Check sheet for the modelled part. Datum: model origin and axes. Units: mm. Coordinates: 2 decimals unless noted, no trailing zeros. Write each loop counter-clockwise with the first axis right and the second up, starting at its lowest first coordinate (ties: lowest second). Pieces come first, ordered by that corner, then holes. Notation, with made-up numbers: (79, 66) -> (92, 66) arc R23 ccw to (92, 77) -> close; hole circle Ø11 at (38, -27.5). An arc over 180 degrees is marked (long way). Put each result on its own line as item: value.
```python
from build123d import *

# Parameters (mm, degrees)
BLOCO_DEPTH            = 9.2
ESBO_O3_W              = 5.6
ESBO_O3_H              = 3.2
RASGO_DO_ENCAIXE_DEPTH = 18.034534118


with BuildPart() as part:
    # Esboço1 → Bloco (new body)
    with BuildSketch(Plane(origin=(0, 0, 0), x_dir=(1, 0, 0), z_dir=(0, 1, 0))):
        with BuildLine():
            Line((0, -75), (0.029321703, -68))
            Line((0.029321703, -68), (-12.770566003, -67.946383642))
            Line((-12.770566003, -67.946383642), (-12.795506441, -73.900439883))
            ThreePointArc((-12.795506441, -73.900439883), (-6.421331979, -74.724604352), (0, -75))
        make_face()
    extrude(amount=BLOCO_DEPTH)

    # Esboço3 → Rasgo do Encaixe (cut, through all)
    with BuildSketch(Plane(origin=(-0.284833888, 0, 67.99868406), x_dir=(-0.9999912270311377, 0, -0.0041887779553967395), z_dir=(0.0041887779553967395, 0, -0.9999912270311377))):
        with Locations((2.485841653, 1.6)):
            Rectangle(ESBO_O3_W, ESBO_O3_H)
    extrude(amount=-RASGO_DO_ENCAIXE_DEPTH, mode=Mode.SUBTRACT)


solid = part.part
```
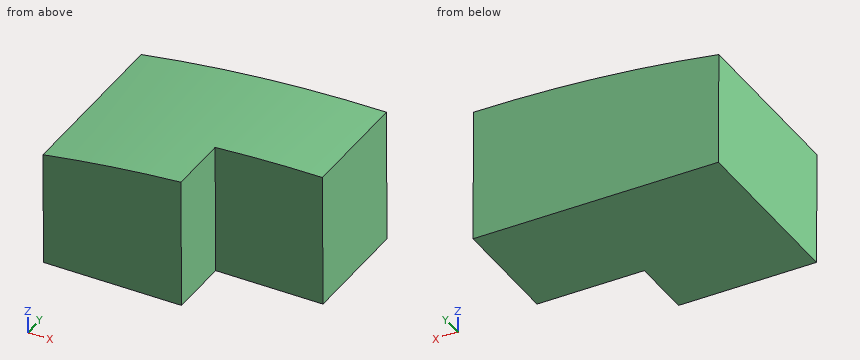
Q1. Cross-section at D-D (z = 70.75). Record the cut outline in (x, y), plus the area to 3 significant figures.
Recorded:
outline: (-12.78, 0) -> (-5.58, 0) -> (-5.58, 3.2) -> (0.02, 3.2) -> (0.02, 9.2) -> (-12.78, 9.2) -> close
area: 99.8 mm2
Q2. Cross-section at C-C (x = -9.25). Record the cut outline in (y, z).
Recorded:
outline: (0, 67.96) -> (9.2, 67.96) -> (9.2, 74.43) -> (0, 74.43) -> close
Q3. Depth check by flat-ended pin: P1, Ø1.7, axis at x = -2.5, z = 70, coming from the -Y side; P2, Ø4, axis at y = 2, z = 74, coming from the +X side; P3, Ø1.5, axis at x = -6, y = 6, coming from the +Z side. Enter the tip coordinate at first touch or a pass-through.
Recorded:
P1: stops at y = 3.2
P2: stops at x = 0.01
P3: stops at z = 74.82
Q4. Material ranges on line 1 along X through (y, z) = (7.5, 68.75); line 2 along Y through (x, z) = (-2.25, 69.25); line 3 along Z through (x, y) = (-9, 1.75), recorded low to high.
Recorded:
line 1: x = -12.77 to 0.03
line 2: y = 3.2 to 9.2
line 3: z = 67.96 to 74.46
Q5. Cross-section at B-B (y = 2.25). Record the cut outline in (x, z).
Recorded:
outline: (-12.8, 73.9) -> (-12.77, 67.95) -> (-5.57, 67.98) -> (-5.6, 74.79) arc R75 ccw to start
Q6. Cross-section at A-A (z = 74.25). Record the cut outline in (x, y).
Recorded:
outline: (-10.58, 0) -> (-5.6, 0) -> (-5.6, 3.2) -> (0, 3.2) -> (0, 9.2) -> (-10.58, 9.2) -> close
